```python
from build123d import *

# Parameters (mm, degrees)
SKETCH_W        = 52.175
SKETCH_H        = 40
PAD_DEPTH       = 7
SKETCH001_R     = 1.85
POCKET_DEPTH    = 2
SKETCH002_R     = 2.4
POCKET001_DEPTH = 3
CHAMFER_SIZE    = 0.7


with BuildPart() as part:
    # Sketch → Pad (new body)
    with BuildSketch(Plane.XY):
        with Locations((-26.0875, 0)):
            Rectangle(SKETCH_W, SKETCH_H)
    extrude(amount=-PAD_DEPTH)

    # Sketch001 → Pocket (cut)
    with BuildSketch(Plane.XY):
        with Locations((-40.005, 13.335)):
            Circle(SKETCH001_R)
        with Locations((-13.335, 13.335)):
            Circle(SKETCH001_R)
        with Locations((-40.005, -13.335)):
            Circle(SKETCH001_R)
        with Locations((-13.335, -13.335)):
            Circle(SKETCH001_R)
    extrude(amount=-POCKET_DEPTH, mode=Mode.SUBTRACT)

    # Sketch002 (on DatumPlane) → Pocket001 (cut)
    with BuildSketch(Plane(origin=(0, 0, -7), x_dir=(-1, 0, 0), z_dir=(0, 0, -1))):
        with Locations((26.0875, 0)):
            Circle(SKETCH002_R)
    extrude(amount=-POCKET001_DEPTH, mode=Mode.SUBTRACT)

    # Chamfer
    chamfer_edges = [part.edges().sort_by_distance(p)[0] for p in [
        (-15.185, -13.335, 0),
        (-41.855, -13.335, 0),
        (-41.855, 13.335, 0),
        (-15.185, 13.335, 0),
    ]]
    chamfer(chamfer_edges, length=CHAMFER_SIZE)


solid = part.part
```
Verification items for the finished model (mm, model axes). A direction names the side the tool comes from. Coordinates: 2 decimals unless noted, no trailing zeros. Write each loop counter-clockwise with the first axis right and the second up, starting at its lowest first coordinate (ties: lowest second). Pieces come first, ordered by that corner, then holes. Notation, with made-up numbers: (-18, 82) - (20, 82) arc R21 ccw to (20, 111) - close; hole circle Ø9 at (6, 73.25). An arc over 180 degrees is marked (long way). One line per question, with ' | ' between items. Start each with the question number.
1. Gauge pin test, flat ends, axial feed: P1, Ø3, axis at x = -26.09, y = 0, coming from the -Z side; P2, Ø1.8, axis at x = -13.5, y = 14, coming from the +Z side. Record the tip position at first contact, or that the pin passes through.
2. Draft check along Y on faces 4 (the flat face through (-26, 0, 0)), 5 (the flat face through (-40, -13, -2)), 6 (the flat face through (-26, -20, -3)). Enter one of: released by +Y, released by -Y, zero draft, split by the parting line, or undercut.
3. Access from +Z, -Z, +X, -X, +Y, -Y to the whole of each face (thin tool, end or side, straight path). Record for faces 1 (the cylindrical face through (-41.369, -12.085, -1.341)), 2 (the flat face through (-26, 0, -4)), 3 (the flat face through (-52.175, 0, -3)).
4. Material ranges on line 1 along X through (y, z) = (-13, -1.75) (3 decimals); line 2 along Y through (x, z) = (-41, -1.75); line 3 along Y through (x, z) = (-28, -5), recorded low to high.
5. Section check B-B (x = -24.5). Enter the section's corners in (y, z).
6. Section check A-A (y = 0). Enter the section's corners in (x, z) (1 decimal), plus the area to 3 significant figures.
Computed values:
1) P1: z = -4 | P2: z = -2
2) face 4: zero draft | face 5: undercut | face 6: released by -Y
3) face 1: +Z | face 2: -Z | face 3: +Z, -Z, -X, +Y, -Y
4) line 1: -52.175 to -41.824, -38.186 to -15.154, -11.516 to 0 | line 2: -20 to -14.89, -11.78 to 11.78, 14.89 to 20 | line 3: -20 to -1.45, 1.45 to 20
5) outline: (-20, -7) - (-1.8, -7) - (-1.8, -4) - (1.8, -4) - (1.8, -7) - (20, -7) - (20, 0) - (-20, 0) - close
6) outline: (-52.2, -7) - (-28.5, -7) - (-28.5, -4) - (-23.7, -4) - (-23.7, -7) - (0, -7) - (0, 0) - (-52.2, 0) - close | area: 351 mm²
